```python
from build123d import *

# Parameters (mm, degrees)
F0_W         = 50.8
F0_H         = 50.8
F1_DEPTH     = 50.8
F2_W         = 40.64
F2_H         = 40.64
F3_DEPTH     = 50.8
F4_W         = 40.64
F4_H         = 40.64
F5_DEPTH     = 50.8
F6_R         = 5.07999
F7_T1_DEPTH  = 58.4224242529
F7_T3_DEPTH  = 58.4224242529
F7_T6_ANGLE  = 90
F7_T8_ANGLE  = 90
F7_T10_ANGLE = 90


# Not quite as in the source:
# - a fillet or chamfer that OpenCascade refuses, or shapes differently, is made with other operations: its cross-section is extruded or revolved along the edge and cut away or added
# - a fillet or chamfer is up to 0.001 mm smaller than in the source, because OpenCascade refuses the exact size


with BuildPart() as f1:
    # F0 (on Front) → F1 (new body)
    with BuildSketch(Plane.XZ):
        with Locations((25.4, 25.4)):
            Rectangle(F0_W, F0_H)
    extrude(amount=F1_DEPTH)

    # F2 (on face) → F3 (cut)
    with BuildSketch(Plane.XZ.offset(50.8)):
        with Locations((25.4, 25.4)):
            Rectangle(F2_W, F2_H)
    extrude(amount=-F3_DEPTH, mode=Mode.SUBTRACT)

    # F4 (on face) → F5 (cut)
    with BuildSketch(Plane.YZ.offset(50.8)):
        with Locations((-25.4, 25.4)):
            Rectangle(F4_W, F4_H)
    extrude(amount=-F5_DEPTH, mode=Mode.SUBTRACT)

    # F6 (radius 5.08 in the source; OpenCascade refuses exactly that, so slightly less here)
    f6_edges = [f1.edges().sort_by_distance(p)[0] for p in [
        (25.4, -50.8, 50.8),
        (50.8, -25.4, 50.8),
        (50.8, -50.8, 25.4),
        (25.4, -50.8, 0),
        (50.8, -25.4, 0),
        (25.4, 0, 0),
        (0, -25.4, 0),
        (50.8, 0, 25.4),
        (25.4, 0, 50.8),
        (0, 0, 25.4),
    ]]
    fillet(f6_edges, radius=F6_R)

    # F7: fillet of radius 5.08 on 3 edges, made by hand

    # F7_s2 → F7_t1 (cut)
    with BuildSketch(Plane.XZ):
        with BuildLine():
            ThreePointArc((-0.0004, 45.7190343146), (1.4878975516, 49.3121024484), (5.0809656854, 50.8004))
            Line((5.0809656854, 50.8004), (5.0809656854, 51.3085365685))
            ThreePointArc((5.0809656854, 51.3085365685), (2.5404828427, 51.3081365685), (0, 51.3081365685))
            Line((0, 51.3081365685), (-0.5081365685, 50.8))
            ThreePointArc((-0.5081365685, 50.8), (-0.5081365685, 48.2595171573), (-0.5085365685, 45.7190343146))
            Line((-0.5085365685, 45.7190343146), (-0.0004, 45.7190343146))
        make_face()
    extrude(amount=F7_T1_DEPTH, mode=Mode.SUBTRACT)

    # F7_s4 → F7_t3 (cut)
    with BuildSketch(Plane.XY):
        with BuildLine():
            ThreePointArc((-0.0004, -45.7190343146), (1.4878975516, -49.3121024484), (5.0809656854, -50.8004))
            Line((5.0809656854, -50.8004), (5.0809656854, -51.3085365685))
            ThreePointArc((5.0809656854, -51.3085365685), (2.5404828427, -51.3081365685), (0, -51.3081365685))
            Line((0, -51.3081365685), (-0.5081365685, -50.8))
            ThreePointArc((-0.5081365685, -50.8), (-0.5081365685, -48.2595171573), (-0.5085365685, -45.7190343146))
            Line((-0.5085365685, -45.7190343146), (-0.0004, -45.7190343146))
        make_face()
    extrude(amount=F7_T3_DEPTH, mode=Mode.SUBTRACT)

    # F7_s5 → F7_t6 (revolve, cut)
    with BuildSketch(Plane.YZ.offset(5.0809656854)):
        with BuildLine():
            ThreePointArc((-45.72041, 0), (-49.3125053774, 1.4878946226), (-50.8004, 5.07999))
            Line((-50.8004, 5.07999), (-50.8004, 0))
            Line((-50.8004, 0), (-45.72041, 0))
        make_face()
    revolve(axis=Axis((5.0809656854, -45.7190343146, 0), (0, 0, -1)), revolution_arc=F7_T6_ANGLE, mode=Mode.SUBTRACT)

    # F7_s7 → F7_t8 (revolve, cut)
    with BuildSketch(Plane.XY.offset(45.7190343146)):
        with BuildLine():
            ThreePointArc((5.07959, 0), (1.4874946226, -1.4878946226), (-0.0004, -5.07999))
            Line((-0.0004, -5.07999), (-0.0004, 0))
            Line((-0.0004, 0), (5.07959, 0))
        make_face()
    revolve(axis=Axis((5.0809656854, 0, 45.7190343146), (0, 1, 0)), revolution_arc=F7_T8_ANGLE, mode=Mode.SUBTRACT)

    # F7_s9 → F7_t10 (revolve, cut)
    with BuildSketch(Plane.XZ.offset(45.72001)):
        with BuildLine():
            ThreePointArc((-0.0003999063, 45.72001), (1.488242525, 49.3124473888), (5.0809656854, 50.8004))
            Line((5.0809656854, 50.8004), (5.0809656854, 51.3085365685))
            ThreePointArc((5.0809656854, 51.3085365685), (2.5404828427, 51.3081365685), (0, 51.3081365685))
            Line((0, 51.3081365685), (-0.5081365685, 50.8))
            Line((-0.5081365685, 50.8), (-0.5085364917, 45.72001))
            Line((-0.5085364917, 45.72001), (-0.0003999063, 45.72001))
        make_face()
    revolve(axis=Axis((0, -45.72001, 45.72001), (1, 0, 0)), revolution_arc=F7_T10_ANGLE, mode=Mode.SUBTRACT)


solid = f1.part
```
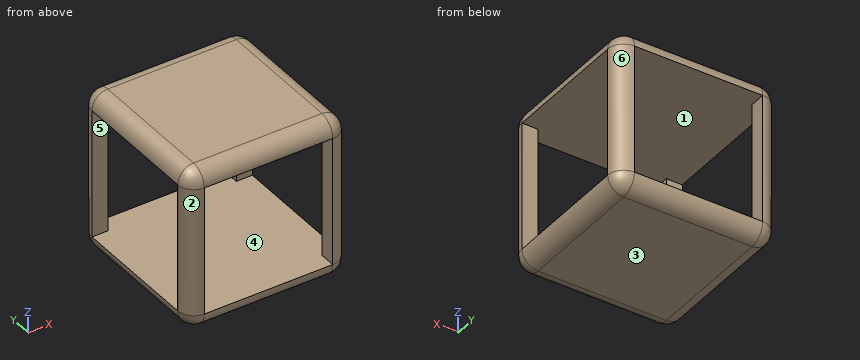
Input: part model. Units: mm. Frame: model coordinates. Face numbers are marked on the shaded views. A direction names the side the tool comes from. Round coordinates to 2 decimals unless told otherwise and drop trailing zeros. One line per item, written item: value.
(1) Mould query, pull axis X, two halves, no side actions, for the marked faces 1, 2, 3 and 4. Classes: pulls with the +X half, pulls with the -X half, needs draft (parallel to the pull), parting line crosses it, or undercut.
Geometry check:
face 1: undercut
face 2: pulls with the -X half
face 3: needs draft
face 4: undercut
(2) Set-up query: the marked faces 5 and 6. Return all of +Z, -Z, +X, -X, +Y, -Y with unobstructed straight access to the full face (end or side cutting, diameter ignored); none if empty.
Geometry check:
face 5: +X, -X
face 6: +Z, -Z, +X, +Y
(3) Material intervals for line 1 (Z direction, x = 9, y = -39); line 2 (X direction, y = -46, z = 21.5); line 3 (Z direction, x = 7, y = -46.5), sorted ascending. Write a range as [from, to].
Geometry check:
line 1: [0, 5.08], [45.72, 50.8]
line 2: [0.01, 5.08], [45.72, 50.79]
line 3: [0.06, 5.08], [45.72, 50.74]
(4) Section C-C (z = 42). Give the number of separate pieces and of enclosed holes in the cut face, plus the area to 3 significant figures.
Geometry check:
separate pieces: 4
enclosed holes: 0
area: 81.1 mm2
(5) Pin query (flat end, axial travel): pin 1 (1.5 mm diameter, centred on y = -2, z = 25, fed in from -X); pin 2 (1.5 mm diameter, centred on y = -1.5, z = 23, fed in from +X); pin 3 (5 mm diameter, centred on y = -10.5, z = 9.5, fed in from +X); pin 4 (1.5 mm diameter, centred on x = 3, z = 27, fed in from -Y). Return the tip coordinate at first contact, or that it passes through.
Geometry check:
pin 1: x = 0.57
pin 2: x = 49.94
pin 3: through
pin 4: y = -50.62
